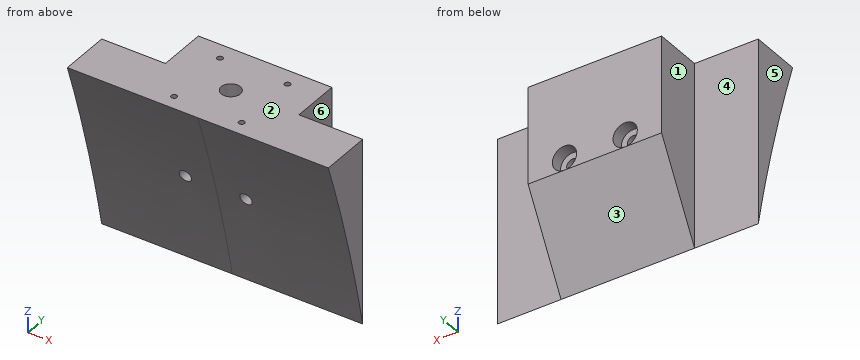
from build123d import *

# Parameters (mm, degrees)
BOSS_EXTRUDE1_DEPTH     = 68.2625
SKETCH4_W               = 69.85
SKETCH4_H               = 25.4
BOSS_EXTRUDE2_DEPTH     = 50.8
CUT_EXTRUDE1_DEPTH      = 364.143790643
CUT_EXTRUDE1_DEPTH_BACK = 364.143790643
SKETCH2_R               = 3.175
SKETCH5_R               = 5
CUT_EXTRUDE2_DEPTH      = 12.7
SKETCH6_R               = 1.5
CUT_EXTRUDE3_DEPTH      = 6.35
CIRPATTERN1_COUNT       = 4
BOSS_EXTRUDE3_DEPTH     = 69.85
SKETCH8_R               = 6.35
CUT_EXTRUDE4_DEPTH      = 6.35


with BuildPart() as part:
    # Sketch1 → Boss-Extrude1 (new, symmetric)
    with BuildSketch(Plane(origin=(0, 0, 0), x_dir=(0, 0, -1), z_dir=(1, 0, 0))):
        with BuildLine():
            Line((-258.749759613, 26.462577976), (-355.687187923, 26.462577976))
            Line((-355.687187923, 26.462577976), (-355.687187923, 0))
            add(Edge.make_bspline(
                [(-355.687187923, 0), (-355.37055154, 0.107976188), (-354.108976481, 0.538185956), (-351.284999827, 1.502859463), (-346.602313416, 3.058862652), (-336.815361237, 6.25189344), (-320.429894612, 11.27779725), (-301.357119069, 16.549630187), (-283.167308194, 21.086195797), (-270.107851124, 24.071552001), (-261.828911243, 25.828285388), (-258.749759613, 26.462577976)],
                knots=[0, 0, 0, 0, 0.001371577, 0.005464776, 0.012234802, 0.021601969, 0.04767125, 0.082496261, 0.102719149, 0.124527079, 0.137415965, 0.137415965, 0.137415965, 0.137415965], degree=3))
        make_face()
    extrude(amount=BOSS_EXTRUDE1_DEPTH, both=True)

    # Sketch4 → Boss-Extrude2 (add)
    with BuildSketch(Plane.XY.offset(355.687187923)):
        with Locations((0, 39.162577976)):
            Rectangle(SKETCH4_W, SKETCH4_H)
    extrude(amount=-BOSS_EXTRUDE2_DEPTH)

    # Sketch2 → Cut-Extrude1 (cut, two sides: drawn at the far end of the back side and taken through both)
    with BuildSketch(Plane(origin=(0, 26.462577976, 0), x_dir=(1, 0, 0), z_dir=(0, 1, 0)).offset(-CUT_EXTRUDE1_DEPTH_BACK)):
        with Locations(Location((-15.875, -311.237187923, 0), (0, 0, 270))):
            Circle(SKETCH2_R)
        with Locations(Location((15.875, -311.237187923, 0), (0, 0, 270))):
            Circle(SKETCH2_R)
    extrude(amount=CUT_EXTRUDE1_DEPTH + CUT_EXTRUDE1_DEPTH_BACK, mode=Mode.SUBTRACT)

    # Sketch5 → Cut-Extrude2 (cut)
    with BuildSketch(Plane.XY.offset(355.687187923)):
        with Locations((0, 25.4)):
            Circle(SKETCH5_R)
    extrude(amount=-CUT_EXTRUDE2_DEPTH, mode=Mode.SUBTRACT)

    # Sketch6 → Cut-Extrude3 (cut)
    with BuildSketch(Plane.XY.offset(355.687187923)):
        with Locations((17.67766953, 43.07766953)):
            Circle(SKETCH6_R)
    cut_extrude3 = extrude(amount=-CUT_EXTRUDE3_DEPTH, mode=Mode.SUBTRACT)

    # CirPattern1: Cut-Extrude3 ×4 about axis
    cirpattern1_axis = Axis((0, 25.4, 0), (0, 0, 1))
    for i in range(1, CIRPATTERN1_COUNT):
        add(cut_extrude3.rotate(cirpattern1_axis, i * 360 / CIRPATTERN1_COUNT), mode=Mode.SUBTRACT)

    # Sketch7 → Boss-Extrude3 (add)
    with BuildSketch(Plane.ZY.offset(34.925)):
        Polygon((304.887187923, 51.862577976), (258.749759613, 26.462577976), (304.887187923, 26.462577976), align=None)
    extrude(amount=-BOSS_EXTRUDE3_DEPTH)

    # Sketch8 → Cut-Extrude4 (cut)
    with BuildSketch(Plane(origin=(0, 51.862577976, 0), x_dir=(1, 0, 0), z_dir=(0, 1, 0))):
        with Locations(Location((15.875, -311.237187923, 0), (0, 0, 270))):
            Circle(SKETCH8_R)
        with Locations(Location((-15.875, -311.237187923, 0), (0, 0, 270))):
            Circle(SKETCH8_R)
    extrude(amount=-CUT_EXTRUDE4_DEPTH, mode=Mode.SUBTRACT)


solid = part.part
Can you work these out from the model? Positions are in its coordinate system, mm. Face numbers are marked on the shaded views. A direction names the side the tool comes from. Give positions to 0.01 mm unless a question says otherwise; leave off trailing zeros. One line per question, with ' | ' between items.
Item 1: We'd pull the mould along Z, two halves only. Please class the marked faces 1, 2 and 3: released by +Z, released by -Z, zero draft, split by the parting line, or undercut.
Answer block:
face 1: zero draft | face 2: released by +Z | face 3: released by -Z
Item 2: Please list where these lines run through material, in increasing order: L1, parallel to X at y = 38, z = 319 (3 decimals); L2, parallel to Y at x = 0, z = 349.5; L3, parallel to Z at x = -14, y = 42.5.
Answer block:
L1: x = -34.925 to 34.925 | L2: y = 2.09 to 20.4, 30.4 to 51.86 | L3: z = 287.88 to 308.67, 313.8 to 355.69
Item 3: I'm going to push flat-ended pins straight in: pin 1 Ø16.5 at (x, z) = (49, 293.5) entering from +Y; pin 2 Ø20.5 at (x, z) = (-15.88, 311.24) entering from -Y; pin 3 Ø7.5 at (y, z) = (34.5, 288) entering from +X (3 decimals); pin 4 Ø11 at (x, y) = (-1.5, 26) entering from +Z. Where does each tip first touch, or does it pass through?
Answer block:
pin 1: stops at y = 26.46 | pin 2: stops at y = 10.86 | pin 3: stops at x = 34.925 | pin 4: stops at z = 355.69
Item 4: For the marked faces 4, 5 and 6, which set-ups out of +Z, -Z, +X, -X, +Y, -Y let a thin tool reach every point of the face, with its end or its side?
Answer block:
face 4: +Z, -Z, -X, +Y | face 5: +Z, -Z, -X, +Y, -Y | face 6: +Z, -Z, +X, +Y
